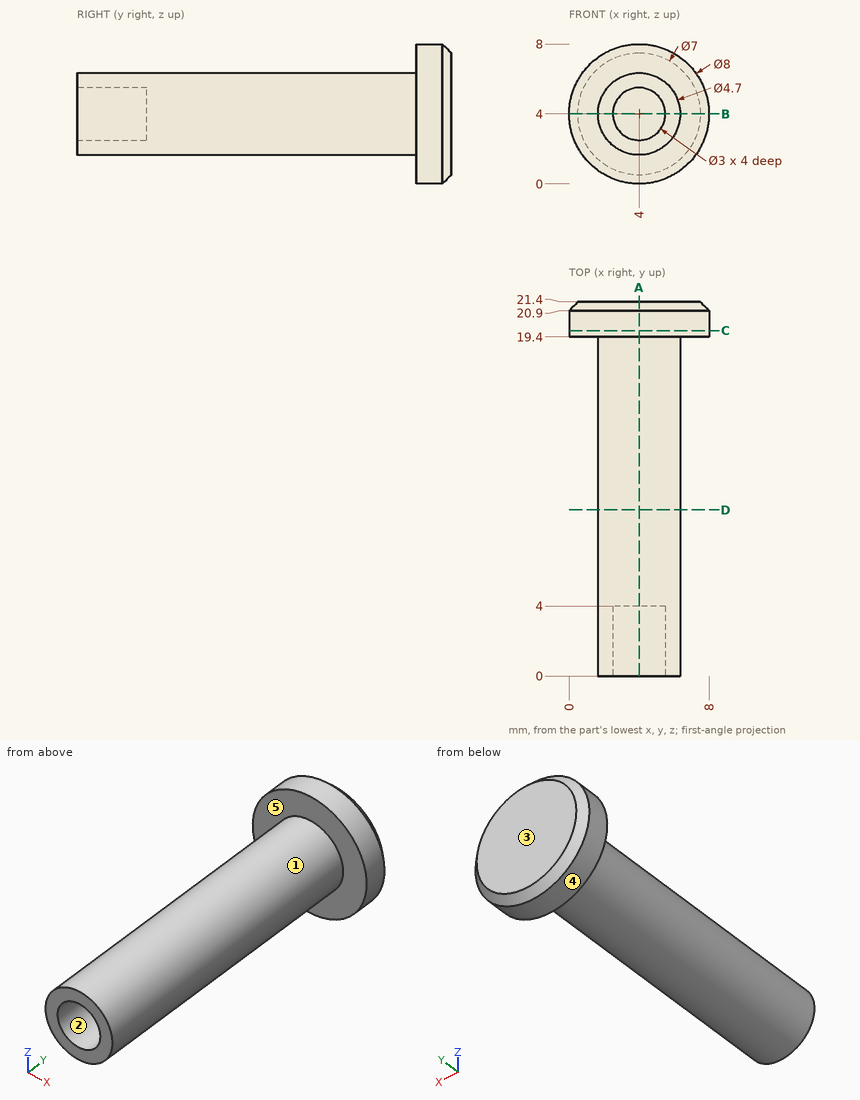
Design review of the part shown in the three views and the two pictorial views. Dimensions are in mm from the part's minimum x, y and z. A direction names the side the tool comes from. Round coordinates to 2 decimals unless told otherwise and drop trailing zeros. Loops run counter-clockwise (first coordinate to the right, second up) from the corner with the lowest first, then second, coordinate; pieces in that order, holes last. Notation, with made-up numbers: M 46.25,-18.5 L 97.25,-18.5 A19 ccw 97.25,16.5 Z; hole C -14,38 d4. An arc over 180 degrees is marked long. Put each result on its own line as item: value.
Q1. For pin 1 (0.9 mm diameter, centred on x = 3.5, z = 3.5, fed in from -Y); pin 2 (1 mm diameter, centred on x = 5, y = 11.5, fed in from -Z), all flat-tipped, find the tip position at first contact; note any pin that passes through.
Result set:
pin 1: stops at y = 4
pin 2: stops at z = 1.7
Q2. Consider section C-C, the plane y = 19.75. Give the boundary of the cut face in (x, z).
Result set:
outline: C 4,4 d8
Q3. To check wall thickness, follow L1, parallel to X at y = 1.05, z = 4; L2, parallel to Y at x = 1, z = 4.75; L3, parallel to Y at x = 4.75, z = 3.25. State the ranges of each line that lie inside material, in increasing order.
Result set:
L1: x = 1.65 to 2.5, 5.5 to 6.35
L2: y = 19.4 to 21.4
L3: y = 4 to 21.4
Q4. Consider section A-A, the plane x = 4. Give the boundary of the cut face in (y, z), then the cut area to 3 significant figures.
Result set:
outline: M 0,1.65 L 19.4,1.65 L 19.4,0 L 20.9,0 L 21.4,0.5 L 21.4,7.5 L 20.9,8 L 19.4,8 L 19.4,6.35 L 0,6.35 L 0,5.5 L 4,5.5 L 4,2.5 L 0,2.5 Z
area: 94.9 mm²
Q5. Consider section B-B, the plane z = 4. Give the boundary of the cut face in (x, y).
Result set:
outline: M 0,19.4 L 1.65,19.4 L 1.65,0 L 2.5,0 L 2.5,4 L 5.5,4 L 5.5,0 L 6.35,0 L 6.35,19.4 L 8,19.4 L 8,20.9 L 7.5,21.4 L 0.5,21.4 L 0,20.9 Z
Q6. Consider section D-D, the plane y = 9.5. Give the boundary of the cut face in (x, z).
Result set:
outline: C 4,4 d4.7
Q7. Machinability: for the marked faces 4 and 5, which of the approach directions +Z, -Z, +X, -X, +Y, -Y give a long, thin tool a straight path to every point of the face, cutting with its end or side? Answer none if there is none.
Result set:
face 4: +Y, -Y
face 5: -Y
Q8. Mouldability with a two-part tool opening along Z and no side actions: class the marked faces 1, 2 and 3 as released by +Z, released by -Z, zero draft, split by the parting line, or undercut.
Result set:
face 1: split by the parting line
face 2: undercut
face 3: zero draft
